Autodesk Inventor part; units mm, degrees
ref_plane "YZ Plane" through (0, 0, 0) normal (1, 0, 0) x (0, 1, 0)
ref_plane "XZ Plane" through (0, 0, 0) normal (0, 1, 0) x (-1, 0, 0)
ref_plane "XY Plane" through (0, 0, 0) normal (0, 0, 1) x (1, 0, 0)
sketch "スケッチ1" plane through (0, 0, 0) normal (0, 0, 1) x (1, 0, 0)
  line L0 (0, 0) -> (260, 0)
  line L1 (260, 0) -> (260, 30)
  line L2 (260, 30) -> (0, 30)
  line L3 (0, 30) -> (0, 0)
  line L4 (0, 15) -> (260, 15)
  circle A0 centre (8, 21) radius 1.6
  circle A1 centre (8, 9) radius 1.6
  circle A2 centre (252, 21) radius 1.6
  circle A3 centre (252, 9) radius 1.6
  point P0 (8, 15)
  point P1 (252, 15)
  dimension "d0" = 260
  dimension "d1" = 244
  dimension "d2" = 8
  dimension "d3" = 30
  dimension "d4" = 15
  dimension "d5" = 9
  dimension "d6" = 9
  dimension "d7" = 9
  dimension "d8" = 9
  dimension "d9" = 3.2
  dimension "d10" = 3.2
  dimension "d11" = 3.2
  dimension "d12" = 3.2
extrude "押し出し1" add sketch "スケッチ1" along normal blind 3
sketch "スケッチ2" plane through (0, 0, 3) normal (0, 0, 1) x (1, 0, 0)
  line L0 (0, 30) -> (0, 0)
  line L1 (0, 0) -> (260, 0)
  line L2 (260, 0) -> (260, 30)
  line L3 (260, 30) -> (0, 30)
  circle A0 centre (8, 9) radius 1.6
  circle A1 centre (252, 9) radius 1.6
  circle A2 centre (252, 21) radius 1.6
  circle A3 centre (8, 21) radius 1.6
  circle A4 centre (8, 21) radius 3
  circle A5 centre (8, 9) radius 3
  circle A6 centre (252, 21) radius 3
  circle A7 centre (252, 9) radius 3
  dimension "d15" = 6
  dimension "d16" = 6
  dimension "d17" = 6
  dimension "d18" = 6
extrude "押し出し2" cut sketch "スケッチ2" against normal blind 1 contours A1 | A4 | A5 | A6 | A7
fillet "フィレット1" radius 2 4 edges at (260, 30, 1.5) (260, 0, 1.5) (0, 30, 1.5) (0, 0, 1.5)
equation "\"d10\" = d9"
equation "\"d11\" = d9"
equation "\"d12\" = d11"
equation "\"d16\" = d15"
equation "\"d17\" = d16"
equation "\"d18\" = d17"
properties part number "BP_BOX-Support-Bar"
Can you work these out from the model? Positions are in its coordinate system, mm. A direction names the side the tool comes from. Round coordinates to 2 decimals unless told otherwise and drop trailing zeros. Answer in a Markdown table with one row per item.
1. I'm going to push flat-ended pins straight in: pin 1 Ø1.8 at (x, y) = (9, 10) entering from +Z; pin 2 Ø2.5 at (x, y) = (252, 9) entering from -Z. Where does each tip first touch, or does it pass through?
Established:
| item | result |
|---|---|
| pin 1 | z = 2 |
| pin 2 | through |
2. Thinking about a two-plate mould opening in X: for faces 3 (the face through (128, 15, 0)), 4 (the face through (249, 21.1, 2.5)), which applies, pulls with the +X half, pulls with the -X half, needs draft (parallel to the pull), parting line crosses it, or undercut?
Established:
| item | result |
|---|---|
| face 3 | needs draft |
| face 4 | undercut |
3. On a 3-axis mill with a long thin cutter (end or side, diameter ignored), from which of +Z, -Z, +X, -X, +Y, -Y can I reach the whole of each face in a straight line? I mean faces 1 (the face through (249, 9.1, 2.5)), 2 (the face through (128, 15, 3)). Say none if no direction works.
Established:
| item | result |
|---|---|
| face 1 | +Z |
| face 2 | +Z, +X, -X, +Y, -Y |
4. Please list where these lines run through material, in increasing order: line 1 (Y direction, x = 8, z = 2.4); line 2 (Y direction, x = 8, z = 1.4); line 3 (X direction, y = 10, z = 1.15). Write a range as from..to.
Established:
| item | result |
|---|---|
| line 1 | 0..6, 12..18, 24..30 |
| line 2 | 0..7.4, 10.6..19.4, 22.6..30 |
| line 3 | 0..6.75, 9.25..250.75, 253.25..260 |
